```python
from build123d import *

# Parameters (mm, degrees)
SKETCH1_W                       = 25
SKETCH1_H                       = 13
BASE_FLANGE1_DEPTH              = 0.9
EDGE_FLANGE1_STRIP_W            = 5.6
EDGE_FLANGE1_STRIP_H            = 0.9
EDGE_FLANGE1_STRIP_CUT_DEPTH    = 80.2
EDGE_FLANGE1_RELIEF_W           = 6.05
EDGE_FLANGE1_RELIEF_H           = 0.45
EDGE_FLANGE1_RELIEF_CUT_DEPTH   = 0.9
EDGE_FLANGE1_STRIP_2_W          = 5.6
EDGE_FLANGE1_STRIP_2_H          = 0.9
EDGE_FLANGE1_STRIP_CUT_2_DEPTH  = 80.2
EDGE_FLANGE1_RELIEF_2_W         = 6.05
EDGE_FLANGE1_RELIEF_2_H         = 0.45
EDGE_FLANGE1_RELIEF_CUT_2_DEPTH = 0.9
EDGE_FLANGE1_STRIP_3_W          = 5.6
EDGE_FLANGE1_STRIP_3_H          = 0.9
EDGE_FLANGE1_STRIP_CUT_3_DEPTH  = 80.2
EDGE_FLANGE1_RELIEF_3_W         = 6.05
EDGE_FLANGE1_RELIEF_3_H         = 0.45
EDGE_FLANGE1_RELIEF_CUT_3_DEPTH = 0.9
EDGE_FLANGE1_STRIP_4_W          = 5.6
EDGE_FLANGE1_STRIP_4_H          = 0.9
EDGE_FLANGE1_STRIP_CUT_4_DEPTH  = 80.2
EDGE_FLANGE1_RELIEF_4_W         = 6.05
EDGE_FLANGE1_RELIEF_4_H         = 0.45
EDGE_FLANGE1_RELIEF_CUT_4_DEPTH = 0.9
EDGE_FLANGE1_DEPTH              = 80.2
EDGE_FLANGE1_BEND_DEPTH         = 80.2
EDGE_FLANGE1_BEND_2_DEPTH       = 80.2
EDGE_FLANGE1_BEND_3_DEPTH       = 80.2
SKETCH18_R                      = 8
CUT_EXTRUDE1_DEPTH              = 10
M2X0_4_TAPPED_HOLE1_D           = 1.6
M2X0_4_TAPPED_HOLE1_DEPTH       = 5.2
M2X0_4_TAPPED_HOLE1_TIP         = 0.480688495
M2X0_4_TAPPED_HOLE2_D           = 1.6
M2X0_4_TAPPED_HOLE2_DEPTH       = 5.2
M2X0_4_TAPPED_HOLE2_TIP         = 0.480688495
M2X0_4_TAPPED_HOLE3_D           = 1.6
M2X0_4_TAPPED_HOLE3_DEPTH       = 5.2
M2X0_4_TAPPED_HOLE3_TIP         = 0.480688495
M2X0_4_TAPPED_HOLE4_D           = 1.6
M2X0_4_TAPPED_HOLE4_DEPTH       = 5.2
M2X0_4_TAPPED_HOLE4_TIP         = 0.480688495
M4_CLEARANCE_HOLE1_D            = 4.5


# Sheet-metal steps are written as plain solids
with BuildPart() as part:
    # Sketch1 → Base-Flange1 (new body)
    with BuildSketch(Plane(origin=(0, 0, 0), x_dir=(1, 0, 0), z_dir=(0, 1, 0))):
        Polygon((9, 98.2), (0, 89.2), (0, 9), (9, 0), (89.2, 0), (98.2, 9), (98.2, 89.2), (89.2, 98.2), align=None)
        with Locations((74.6, 48.2)):
            Rectangle(SKETCH1_W, SKETCH1_H, mode=Mode.SUBTRACT)
        with Locations((23.6, 48.2)):
            Rectangle(SKETCH1_W, SKETCH1_H, mode=Mode.SUBTRACT)
    extrude(amount=-BASE_FLANGE1_DEPTH)

    # Edge-Flange1 strip (across the edge) → Edge-Flange1 strip cut (cut)
    with BuildSketch(Plane(origin=(98.2, -0.9, -89.2), x_dir=(-1, 0, 0), z_dir=(0, 0, 1))):
        with Locations((-0.9, -0.45)):
            Rectangle(EDGE_FLANGE1_STRIP_W, EDGE_FLANGE1_STRIP_H)
    extrude(amount=EDGE_FLANGE1_STRIP_CUT_DEPTH, mode=Mode.SUBTRACT)

    # Edge-Flange1 relief (on the sheet) → Edge-Flange1 relief cut (cut)
    with BuildSketch(Plane(origin=(96.3, -0.9, -89.2), x_dir=(-1, 0, 0), z_dir=(0, -1, 0))):
        with Locations((-2.575, 0.225)):
            Rectangle(EDGE_FLANGE1_RELIEF_W, EDGE_FLANGE1_RELIEF_H)
        with Locations((-2.575, -80.425)):
            Rectangle(EDGE_FLANGE1_RELIEF_W, EDGE_FLANGE1_RELIEF_H)
    extrude(amount=-EDGE_FLANGE1_RELIEF_CUT_DEPTH, mode=Mode.SUBTRACT)

    # Edge-Flange1 strip 2 (across the edge) → Edge-Flange1 strip cut 2 (cut)
    with BuildSketch(Plane(origin=(89.2, -0.9, 0), x_dir=(0, 0, -1), z_dir=(-1, 0, 0))):
        with Locations((-0.9, -0.45)):
            Rectangle(EDGE_FLANGE1_STRIP_2_W, EDGE_FLANGE1_STRIP_2_H)
    extrude(amount=EDGE_FLANGE1_STRIP_CUT_2_DEPTH, mode=Mode.SUBTRACT)

    # Edge-Flange1 relief 2 (on the sheet) → Edge-Flange1 relief cut 2 (cut)
    with BuildSketch(Plane(origin=(89.2, -0.9, -1.9), x_dir=(0, 0, -1), z_dir=(0, -1, 0))):
        with Locations((-2.575, 0.225)):
            Rectangle(EDGE_FLANGE1_RELIEF_2_W, EDGE_FLANGE1_RELIEF_2_H)
        with Locations((-2.575, -80.425)):
            Rectangle(EDGE_FLANGE1_RELIEF_2_W, EDGE_FLANGE1_RELIEF_2_H)
    extrude(amount=-EDGE_FLANGE1_RELIEF_CUT_2_DEPTH, mode=Mode.SUBTRACT)

    # Edge-Flange1 strip 3 (across the edge) → Edge-Flange1 strip cut 3 (cut)
    with BuildSketch(Plane(origin=(0, -0.9, -9), x_dir=(1, 0, 0), z_dir=(0, 0, -1))):
        with Locations((-0.9, -0.45)):
            Rectangle(EDGE_FLANGE1_STRIP_3_W, EDGE_FLANGE1_STRIP_3_H)
    extrude(amount=EDGE_FLANGE1_STRIP_CUT_3_DEPTH, mode=Mode.SUBTRACT)

    # Edge-Flange1 relief 3 (on the sheet) → Edge-Flange1 relief cut 3 (cut)
    with BuildSketch(Plane(origin=(1.9, -0.9, -9), x_dir=(1, 0, 0), z_dir=(0, -1, 0))):
        with Locations((-2.575, 0.225)):
            Rectangle(EDGE_FLANGE1_RELIEF_3_W, EDGE_FLANGE1_RELIEF_3_H)
        with Locations((-2.575, -80.425)):
            Rectangle(EDGE_FLANGE1_RELIEF_3_W, EDGE_FLANGE1_RELIEF_3_H)
    extrude(amount=-EDGE_FLANGE1_RELIEF_CUT_3_DEPTH, mode=Mode.SUBTRACT)

    # Edge-Flange1 strip 4 (across the edge) → Edge-Flange1 strip cut 4 (cut)
    with BuildSketch(Plane(origin=(9, -0.9, -98.2), x_dir=(0, 0, 1), z_dir=(1, 0, 0))):
        with Locations((-0.9, -0.45)):
            Rectangle(EDGE_FLANGE1_STRIP_4_W, EDGE_FLANGE1_STRIP_4_H)
    extrude(amount=EDGE_FLANGE1_STRIP_CUT_4_DEPTH, mode=Mode.SUBTRACT)

    # Edge-Flange1 relief 4 (on the sheet) → Edge-Flange1 relief cut 4 (cut)
    with BuildSketch(Plane(origin=(9, -0.9, -96.3), x_dir=(0, 0, 1), z_dir=(0, -1, 0))):
        with Locations((-2.575, 0.225)):
            Rectangle(EDGE_FLANGE1_RELIEF_4_W, EDGE_FLANGE1_RELIEF_4_H)
        with Locations((-2.575, -80.425)):
            Rectangle(EDGE_FLANGE1_RELIEF_4_W, EDGE_FLANGE1_RELIEF_4_H)
    extrude(amount=-EDGE_FLANGE1_RELIEF_CUT_4_DEPTH, mode=Mode.SUBTRACT)

    # Edge-Flange1 section (across the edge) → Edge-Flange1 (add)
    with BuildSketch(Plane(origin=(98.2, -0.9, -89.2), x_dir=(-1, 0, 0), z_dir=(0, 0, 1))):
        with BuildLine():
            Line((0, 1), (0, 9.1))
            Line((0, 9.1), (0.9, 9.1))
            Line((0.9, 9.1), (0.9, 1))
            ThreePointArc((0.9, 1), (1.192893219, 0.292893219), (1.9, 0))
            Line((1.9, 0), (1.9, -0.9))
            ThreePointArc((1.9, -0.9), (0.556497116, -0.343502884), (0, 1))
        make_face()
    extrude(amount=EDGE_FLANGE1_DEPTH)

    # Edge-Flange1 section 2 (across the edge) → Edge-Flange1 bend (add)
    with BuildSketch(Plane(origin=(89.2, -0.9, 0), x_dir=(0, 0, -1), z_dir=(-1, 0, 0))):
        with BuildLine():
            Line((0, 1), (0, 9.1))
            Line((0, 9.1), (0.9, 9.1))
            Line((0.9, 9.1), (0.9, 1))
            ThreePointArc((0.9, 1), (1.192893219, 0.292893219), (1.9, 0))
            Line((1.9, 0), (1.9, -0.9))
            ThreePointArc((1.9, -0.9), (0.556497116, -0.343502884), (0, 1))
        make_face()
    extrude(amount=EDGE_FLANGE1_BEND_DEPTH)

    # Edge-Flange1 section 3 (across the edge) → Edge-Flange1 bend 2 (add)
    with BuildSketch(Plane(origin=(0, -0.9, -9), x_dir=(1, 0, 0), z_dir=(0, 0, -1))):
        with BuildLine():
            Line((0, 1), (0, 9.1))
            Line((0, 9.1), (0.9, 9.1))
            Line((0.9, 9.1), (0.9, 1))
            ThreePointArc((0.9, 1), (1.192893219, 0.292893219), (1.9, 0))
            Line((1.9, 0), (1.9, -0.9))
            ThreePointArc((1.9, -0.9), (0.556497116, -0.343502884), (0, 1))
        make_face()
    extrude(amount=EDGE_FLANGE1_BEND_2_DEPTH)

    # Edge-Flange1 section 4 (across the edge) → Edge-Flange1 bend 3 (add)
    with BuildSketch(Plane(origin=(9, -0.9, -98.2), x_dir=(0, 0, 1), z_dir=(1, 0, 0))):
        with BuildLine():
            Line((0, 1), (0, 9.1))
            Line((0, 9.1), (0.9, 9.1))
            Line((0.9, 9.1), (0.9, 1))
            ThreePointArc((0.9, 1), (1.192893219, 0.292893219), (1.9, 0))
            Line((1.9, 0), (1.9, -0.9))
            ThreePointArc((1.9, -0.9), (0.556497116, -0.343502884), (0, 1))
        make_face()
    extrude(amount=EDGE_FLANGE1_BEND_3_DEPTH)

    # Sketch18 → Cut-Extrude1 (cut)
    with BuildSketch(Plane(origin=(0, 0, 0), x_dir=(1, 0, 0), z_dir=(0, 1, 0))):
        with Locations(Location((49.1, 23.9, 0), (0, 0, 270))):
            Circle(SKETCH18_R)
        with BuildLine():
            Line((11.1, 69.7), (11.1, 71.3))
            ThreePointArc((11.1, 71.3), (15.493398282, 81.906601718), (26.1, 86.3))
            Line((26.1, 86.3), (36.1, 86.3))
            ThreePointArc((36.1, 86.3), (39.635533906, 84.835533906), (41.1, 81.3))
            Line((41.1, 81.3), (41.1, 69.7))
            ThreePointArc((41.1, 69.7), (39.635533906, 66.164466094), (36.1, 64.7))
            Line((36.1, 64.7), (16.1, 64.7))
            ThreePointArc((16.1, 64.7), (12.564466094, 66.164466094), (11.1, 69.7))
        make_face()
        with BuildLine():
            Line((62.1, 64.7), (82.1, 64.7))
            ThreePointArc((82.1, 64.7), (85.635533906, 66.164466094), (87.1, 69.7))
            Line((87.1, 69.7), (87.1, 71.3))
            ThreePointArc((87.1, 71.3), (82.706601718, 81.906601718), (72.1, 86.3))
            Line((72.1, 86.3), (62.1, 86.3))
            ThreePointArc((62.1, 86.3), (58.564466094, 84.835533906), (57.1, 81.3))
            Line((57.1, 81.3), (57.1, 69.7))
            ThreePointArc((57.1, 69.7), (58.564466094, 66.164466094), (62.1, 64.7))
        make_face()
    extrude(amount=-CUT_EXTRUDE1_DEPTH, mode=Mode.SUBTRACT)

    # M2x0.4 Tapped Hole1
    with Locations(Plane(origin=(102.384287404, -9.723815531, 0), x_dir=(1, 0, 0), z_dir=(0, 0, 1))):
        with Locations((-83.284287404, 5.473815531), (-53.284287404, 5.473815531), (-23.284287404, 5.473815531)):
            Hole(M2X0_4_TAPPED_HOLE1_D / 2, depth=M2X0_4_TAPPED_HOLE1_DEPTH)
            with Locations((0, 0, -(M2X0_4_TAPPED_HOLE1_DEPTH + M2X0_4_TAPPED_HOLE1_TIP / 2))):  # 118° drill point
                Cone(0, M2X0_4_TAPPED_HOLE1_D / 2, M2X0_4_TAPPED_HOLE1_TIP, mode=Mode.SUBTRACT)

    # M2x0.4 Tapped Hole2
    with Locations(Plane(origin=(0, -9.723815531, -74.008101688), x_dir=(0, 0, 1), z_dir=(-1, 0, 0))):
        with Locations((54.908101688, 5.473815531), (24.908101688, 5.473815531), (-5.091898312, 5.473815531)):
            Hole(M2X0_4_TAPPED_HOLE2_D / 2, depth=M2X0_4_TAPPED_HOLE2_DEPTH)
            with Locations((0, 0, -(M2X0_4_TAPPED_HOLE2_DEPTH + M2X0_4_TAPPED_HOLE2_TIP / 2))):  # 118° drill point
                Cone(0, M2X0_4_TAPPED_HOLE2_D / 2, M2X0_4_TAPPED_HOLE2_TIP, mode=Mode.SUBTRACT)

    # M2x0.4 Tapped Hole3
    with Locations(Plane(origin=(102.384287404, -9.723815531, -98.2), x_dir=(-1, 0, 0), z_dir=(0, 0, -1))):
        with Locations((23.284287404, 5.473815531), (53.284287404, 5.473815531), (83.284287404, 5.473815531)):
            Hole(M2X0_4_TAPPED_HOLE3_D / 2, depth=M2X0_4_TAPPED_HOLE3_DEPTH)
            with Locations((0, 0, -(M2X0_4_TAPPED_HOLE3_DEPTH + M2X0_4_TAPPED_HOLE3_TIP / 2))):  # 118° drill point
                Cone(0, M2X0_4_TAPPED_HOLE3_D / 2, M2X0_4_TAPPED_HOLE3_TIP, mode=Mode.SUBTRACT)

    # M2x0.4 Tapped Hole4
    with Locations(Plane(origin=(98.2, -9.723815531, -74.008101688), x_dir=(0, 0, -1), z_dir=(1, 0, 0))):
        with Locations((-24.908101688, 5.473815531), (5.091898312, 5.473815531), (-54.908101688, 5.473815531)):
            Hole(M2X0_4_TAPPED_HOLE4_D / 2, depth=M2X0_4_TAPPED_HOLE4_DEPTH)
            with Locations((0, 0, -(M2X0_4_TAPPED_HOLE4_DEPTH + M2X0_4_TAPPED_HOLE4_TIP / 2))):  # 118° drill point
                Cone(0, M2X0_4_TAPPED_HOLE4_D / 2, M2X0_4_TAPPED_HOLE4_TIP, mode=Mode.SUBTRACT)

    # M4 Clearance Hole1 (through all)
    with Locations(Plane(origin=(102.384287404, 0, -74.008101688), x_dir=(1, 0, 0), z_dir=(0, 1, 0))):
        with Locations((-92.284287404, 14.091898312), (-92.284287404, -63.908101688), (-14.284287404, -63.908101688), (-14.284287404, 14.091898312)):
            Hole(M4_CLEARANCE_HOLE1_D / 2)


solid = part.part
```
Check sheet for the modelled part. Datum: model origin and axes. Units: mm. A direction names the side the tool comes from. Coordinates: 2 decimals unless noted, no trailing zeros. Order: outer loops, then holes, each group sorted by start corner. A loop starts at its lowest first (then second) coordinate and runs counter-clockwise, first axis right, second up. Notation, with made-up numbers: M 23,4 L 47,4 A33 cw 47,40 Z; hole C 83.5,-34 d10. An arc over 180 degrees is marked long. Write each question's results on one line, items separated by ' | '. Start each with the question number.
1. Go/stop test with flat-tipped pins: P1, Ø2.5, axis at y = -3.5, z = -97, coming from the -X side; P2, Ø8, axis at x = 43, z = -67, coming from the -Y side; P3, Ø9.5, axis at x = 49.1, z = -23.9, coming from the -Y side; P4, Ø1, axis at y = -0.5, z = -77.5, coming from the +X side. Record where each tip stops, or that it passes through.
2. Material ranges on probe 1 along Z at (x, y) = (44.5, -3.5); probe 2 along X at (y, z) = (-4.5, -46); probe 3 along Z at (x, y) = (10.1, -0.5), recorded low to high.
3. Cross-section at B-B on y = -8.5. Record the cut outline in (x, z), and give its area (3 significant figures).
4. Cross-section at D-D on x = 14. Record the cut outline in (y, z), and give its area (3 significant figures).
5. Cross-section at A-A on z = -53. Record the cut outline in (x, y).
6. Access from +Z, -Z, +X, -X, +Y, -Y to the whole of each face (thin tool, end or side, straight path). Record for faces 5 (the face through (9, -4, -0.7)), 6 (the face through (58.53, -0.44, -66.2)), 7 (the face through (0.7, -4, -9)).
7. Mould release check, pull along Z, two halves, no side actions. Record for faces 1 (the face through (39.67, -0.44, -66.2)), 2 (the face through (49, -6, -98.2)), 3 (the face through (0, -6, -49)), 4 (the face through (50, -6, 0)): +Z half, -Z half, draft (parallel to the pull), parting line (faces both ways), or undercut.
8. Cross-section at C-C on z = -23.9. Record the cut outline in (x, y).
Checks:
1) P1: stops at x = 9 | P2: stops at y = -0.9 | P3: passes through | P4: stops at x = 97.97
2) probe 1: z = -98.2 to -97.3, -0.9 to 0 | probe 2: x = 0 to 0.9, 97.3 to 98.2 | probe 3: z = -97.58 to -90.35, -85.85 to -12.35, -7.85 to -0.62
3) outline: M 0,-89.2 L 0.9,-89.2 L 0.9,-9 L 0,-9 Z; M 9,-98.2 L 89.2,-98.2 L 89.2,-97.3 L 9,-97.3 Z; M 9,-0.9 L 89.2,-0.9 L 89.2,0 L 9,0 Z; M 97.3,-89.2 L 98.2,-89.2 L 98.2,-9 L 97.3,-9 Z | area: 289 mm²
4) outline: M -10,-98.2 L -1.9,-98.2 A1.9 ccw 0,-96.3 L 0,-80.17 L -0.9,-80.17 L -0.9,-96.3 A1 cw -1.9,-97.3 L -10,-97.3 Z; M -10,-0.9 L -1.9,-0.9 A1 cw -0.9,-1.9 L -0.9,-41.7 L 0,-41.7 L 0,-1.9 A1.9 ccw -1.9,0 L -10,0 Z; M -0.9,-65.16 L 0,-65.16 L 0,-54.7 L -0.9,-54.7 Z | area: 78.4 mm²
5) outline: M 0,-10 L 0.9,-10 L 0.9,-1.9 A1 cw 1.9,-0.9 L 11.1,-0.9 L 11.1,0 L 1.9,0 A1.9 ccw 0,-1.9 Z; M 36.1,-0.9 L 62.1,-0.9 L 62.1,0 L 36.1,0 Z; M 87.1,-0.9 L 96.3,-0.9 A1 cw 97.3,-1.9 L 97.3,-10 L 98.2,-10 L 98.2,-1.9 A1.9 ccw 96.3,0 L 87.1,0 Z
6) face 5: +Z, +Y, -Y | face 6: +Y, -Y | face 7: -X, +Y, -Y
7) face 1: undercut | face 2: -Z half | face 3: draft | face 4: +Z half
8) outline: M 0,-10 L 0.9,-10 L 0.9,-1.9 A1 cw 1.9,-0.9 L 41.1,-0.9 L 41.1,0 L 1.9,0 A1.9 ccw 0,-1.9 Z; M 57.1,-0.9 L 96.3,-0.9 A1 cw 97.3,-1.9 L 97.3,-10 L 98.2,-10 L 98.2,-1.9 A1.9 ccw 96.3,0 L 57.1,0 Z
